CAD build for the part. Positions are in the model's coordinates, mm. Face numbers are marked on the shaded views. Give positions to 0.01 mm unless a question says otherwise; leave off trailing zeros. Order: outer loops, then holes, each group sorted by start corner. A loop starts at its lowest first (then second) coordinate and runs counter-clockwise, first axis right, second up. Notation, with made-up numbers: M 64,62.5 L 95,62.5 A22 ccw 95,90.5 Z; hole C -28.75,47.25 d9. An arc over 180 degrees is marked long. Put each result on its own line as item: value. Start each with the question number.
1) Pin check, flat tips, straight feed: pin 1 (5 mm diameter, centred on x = -118.5, y = -15.5, fed in from +Z); pin 2 (1.6 mm diameter, centred on x = -149, y = 14.5, fed in from -Z); pin 3 (4.5 mm diameter, centred on x = -152, y = -4, fed in from +Z). Stop position of each tip, or through.
2) Cut at C-C (x = -134). Write the cut outline in (y, z), and give its area (3 significant figures).
3) Cut at B-B (z = -58). Write the cut outline in (x, y), and give its area (3 significant figures).
4) Drill centre lines: line 1 (Y direction, x = -118.5, z = -65.1); line 2 (Y direction, x = -118, z = -65); line 3 (X direction, y = -1, z = -60). Where is each one in solid material? Low to high. Write a range as [from, to].
5) Two-plate mould, pull along X, no slides. Class the marked faces 1, 2, 3 and 4: released by +X, released by -X, zero draft, split by the parting line, or undercut.
6) Cut at A-A (y = -11). Write the cut outline in (x, z).
7) Cut at D-D (z = -25.5). Write the cut outline in (x, y), and give its area (3 significant figures).
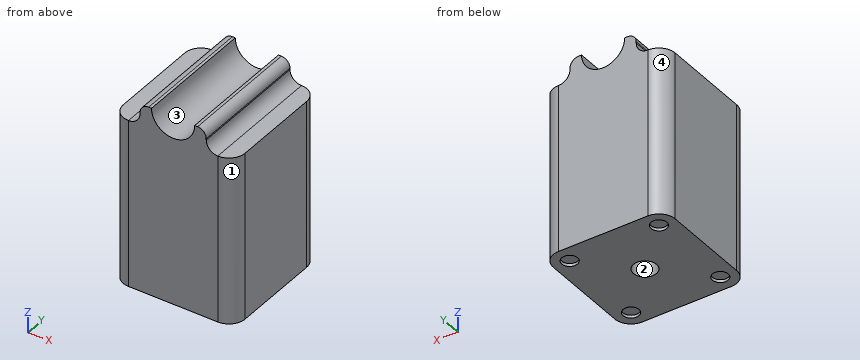
```python
from build123d import *

# Parameters (mm, degrees)
SKETCH047_W     = 42.3
SKETCH047_H     = 42.3
SKETCH047_R     = 4
PAD021_DEPTH    = 12.7
SKETCH053_W     = 42.3
SKETCH053_H     = 42.3
SKETCH054_W     = 42.3
SKETCH054_H     = 42.3
SKETCH055_W     = 23
SKETCH055_H     = 42.3
PAD022_DEPTH    = 7.5
SKETCH056_R     = 7.5
POCKET008_DEPTH = 50
SKETCH048_R     = 2.75
POCKET009_DEPTH = 1
FILLET007_R     = 4
FILLET008_R     = 3
FILLET009_R     = 5.6


with BuildPart() as part:
    # Sketch047 (on Face1 of Binder017) → Pad021 (new body)
    with BuildSketch(Plane.XY.offset(-65.702215)):
        with Locations((-134, 0)):
            Rectangle(SKETCH047_W, SKETCH047_H)
        with Locations((-134, 0)):
            Circle(SKETCH047_R, mode=Mode.SUBTRACT)
    extrude(amount=PAD021_DEPTH)

    # Sketch053 → AdditiveLoft004 section 0
    with BuildSketch(Plane.XY.offset(-53.002215)):
        with Locations((-134, 0)):
            Rectangle(SKETCH053_W, SKETCH053_H)
    # Sketch054 (on DatumPlane) → AdditiveLoft004 section 1
    with BuildSketch(Plane.XY.offset(-7.5)):
        with Locations((-134, 0)):
            Rectangle(SKETCH054_W, SKETCH054_H)
    loft()

    # Sketch055 (on Face10 of AdditiveLoft004) → Pad022 (join)
    with BuildSketch(Plane.XY.offset(-7.5)):
        with Locations((-134, 0)):
            Rectangle(SKETCH055_W, SKETCH055_H)
    extrude(amount=PAD022_DEPTH)

    # Sketch056 (on Face18 of Pad022) → Pocket008 (cut)
    with BuildSketch(Plane.XZ.offset(21.15)):
        with Locations((-134, 0)):
            Circle(SKETCH056_R)
    extrude(amount=-POCKET008_DEPTH, mode=Mode.SUBTRACT)

    # Sketch048 (on Face1 of Binder017) → Pocket009 (cut)
    with BuildSketch(Plane.XY.offset(-65.702215)):
        with Locations((-149.5, -15.5)):
            Circle(SKETCH048_R)
        with Locations((-118.5, -15.5)):
            Circle(SKETCH048_R)
        with Locations((-118.5, 15.5)):
            Circle(SKETCH048_R)
        with Locations((-149.5, 15.5)):
            Circle(SKETCH048_R)
    extrude(amount=POCKET009_DEPTH, mode=Mode.SUBTRACT)

    # Fillet007
    fillet007_edges = [part.edges().sort_by_distance(p)[0] for p in [
        (-122.5, 0, -7.5),
        (-145.5, 0, -7.5),
    ]]
    fillet(fillet007_edges, radius=FILLET007_R)

    # Fillet008
    fillet008_edges = [part.edges().sort_by_distance(p)[0] for p in [
        (-122.5, 0, 0),
        (-145.5, 0, 0),
    ]]
    fillet(fillet008_edges, radius=FILLET008_R)

    # Fillet009
    fillet009_edges = [part.edges().sort_by_distance(p)[0] for p in [
        (-155.15, -21.15, -30.251107),
        (-155.15, -21.15, -59.352215),
        (-155.15, 21.15, -30.251107),
        (-155.15, 21.15, -59.352215),
        (-112.85, -21.15, -30.251107),
        (-112.85, -21.15, -59.352215),
        (-112.85, 21.15, -59.352215),
        (-112.85, 21.15, -30.251107),
    ]]
    fillet(fillet009_edges, radius=FILLET009_R)


solid = part.part
```
Solution:
1. pin 1: z = -6.62
1. pin 2: z = -64.7
1. pin 3: z = -7.5
2. outline: M -21.15,-65.7 L -4,-65.7 L -4,-53 L 4,-53 L 4,-65.7 L 21.15,-65.7 L 21.15,-7.5 L -21.15,-7.5 Z
2. area: 2,360 mm²
3. outline: M -155.15,-15.55 A5.6 ccw -149.55,-21.15 L -118.45,-21.15 A5.6 ccw -112.85,-15.55 L -112.85,15.55 A5.6 ccw -118.45,21.15 L -149.55,21.15 A5.6 ccw -155.15,15.55 Z; hole C -134,0 d8
3. area: 1,710 mm²
4. line 1: [-21.15, -18.25], [-12.75, 12.75], [18.25, 21.15]
4. line 2: [-21.13, -18.2], [-12.8, 12.8], [18.2, 21.13]
4. line 3: [-155.15, -137.87], [-130.13, -112.85]
5. face 1: released by +X
5. face 2: undercut
5. face 3: undercut
5. face 4: released by -X
6. outline: M -155.15,-65.7 L -112.85,-65.7 L -112.85,-7.5 L -118.5,-7.5 A4 cw -122.5,-3.5 L -122.5,-3 A3 ccw -125.5,0 L -126.5,0 A7.5 cw -141.5,0 L -142.5,0 A3 ccw -145.5,-3 L -145.5,-3.5 A4 cw -149.5,-7.5 L -155.15,-7.5 Z
7. outline: M -155.15,-15.55 A5.6 ccw -149.55,-21.15 L -118.45,-21.15 A5.6 ccw -112.85,-15.55 L -112.85,15.55 A5.6 ccw -118.45,21.15 L -149.55,21.15 A5.6 ccw -155.15,15.55 Z
7. area: 1,760 mm²
